The listing builds one solid part. Answer for the finished solid, in the listing's coordinates (mm). A direction names the side the tool comes from. Coordinates: 2 decimals unless noted, no trailing zeros. Order: outer loops, then holes, each group sorted by start corner. A loop starts at its lowest first (then second) coordinate and runs counter-clockwise, first axis right, second up. Notation, with made-up numbers: (-12.5, -8) -> (40.5, -8) arc R22 ccw to (40.5, 18) -> close; hole circle Ø4 at (52.5, -10.5). An arc over 180 degrees is marked (long way). Return JSON: item names as keys, results as strings.
```python
from build123d import *

# Parameters (mm, degrees)
SKETCH1_W           = 300
SKETCH1_H           = 300
SKETCH1_W_2         = 287.3
SKETCH1_H_2         = 287.3
BOSS_EXTRUDE1_DEPTH = 39.8272
CUT_EXTRUDE1_REACH  = 339.766
SKETCH3_W           = 9.414604459
SKETCH3_H           = 11.065164
SKETCH3_W_2         = 16.002
SKETCH3_H_2         = 13.335
SKETCH3_W_3         = 15.3
SKETCH3_H_3         = 12.7
SKETCH3_W_4         = 9
SKETCH3_H_4         = 11


with BuildPart() as part:
    # Sketch1 → Boss-Extrude1 (new body)
    with BuildSketch(Plane(origin=(0, 0, 0), x_dir=(1, 0, 0), z_dir=(0, 1, 0))):
        Rectangle(SKETCH1_W, SKETCH1_H)
        Rectangle(SKETCH1_W_2, SKETCH1_H_2, mode=Mode.SUBTRACT)
    extrude(amount=BOSS_EXTRUDE1_DEPTH)

    # Sketch3 → Cut-Extrude1 (cut, up to next)
    with BuildSketch(Plane(origin=(0, 0, -150), x_dir=(-1, 0, 0), z_dir=(0, 0, -1)), mode=Mode.PRIVATE) as cut_extrude1_sk1:
        with Locations((-111.859321897, 7.773371258)):
            Rectangle(SKETCH3_W, SKETCH3_H)
    cut_extrude1_tool1 = extrude(cut_extrude1_sk1.sketch, amount=-CUT_EXTRUDE1_REACH, mode=Mode.PRIVATE) & part.part
    # Sketch3 → Cut-Extrude1 (cut, up to next)
    with BuildSketch(Plane(origin=(0, 0, -150), x_dir=(-1, 0, 0), z_dir=(0, 0, -1)), mode=Mode.PRIVATE) as cut_extrude1_sk2:
        with Locations((-91.547624126, 6.5913)):
            Rectangle(SKETCH3_W_2, SKETCH3_H_2)
    cut_extrude1_tool2 = extrude(cut_extrude1_sk2.sketch, amount=-CUT_EXTRUDE1_REACH, mode=Mode.PRIVATE) & part.part
    # Sketch3 → Cut-Extrude1 (cut, up to next)
    with BuildSketch(Plane(origin=(0, 0, -150), x_dir=(-1, 0, 0), z_dir=(0, 0, -1)), mode=Mode.PRIVATE) as cut_extrude1_sk3:
        with Locations((-38.618448478, 7.9248)):
            Rectangle(SKETCH3_W_3, SKETCH3_H_3)
    cut_extrude1_tool3 = extrude(cut_extrude1_sk3.sketch, amount=-CUT_EXTRUDE1_REACH, mode=Mode.PRIVATE) & part.part
    # Sketch3 → Cut-Extrude1 (cut, up to next)
    with BuildSketch(Plane(origin=(0, 0, -150), x_dir=(-1, 0, 0), z_dir=(0, 0, -1)), mode=Mode.PRIVATE) as cut_extrude1_sk4:
        with Locations((-18.092571078, 7.9248)):
            Rectangle(SKETCH3_W_3, SKETCH3_H_3)
    cut_extrude1_tool4 = extrude(cut_extrude1_sk4.sketch, amount=-CUT_EXTRUDE1_REACH, mode=Mode.PRIVATE) & part.part
    # Sketch3 → Cut-Extrude1 (cut, up to next)
    with BuildSketch(Plane(origin=(0, 0, -150), x_dir=(-1, 0, 0), z_dir=(0, 0, -1)), mode=Mode.PRIVATE) as cut_extrude1_sk5:
        with Locations((6.757428922, 7.1748)):
            Rectangle(SKETCH3_W_4, SKETCH3_H_4)
    cut_extrude1_tool5 = extrude(cut_extrude1_sk5.sketch, amount=-CUT_EXTRUDE1_REACH, mode=Mode.PRIVATE) & part.part
    # Sketch3 → Cut-Extrude1 (cut, up to next)
    with BuildSketch(Plane(origin=(0, 0, -150), x_dir=(-1, 0, 0), z_dir=(0, 0, -1)), mode=Mode.PRIVATE) as cut_extrude1_sk6:
        with Locations((28.457428922, 7.1748)):
            Rectangle(SKETCH3_W_4, SKETCH3_H_4)
    cut_extrude1_tool6 = extrude(cut_extrude1_sk6.sketch, amount=-CUT_EXTRUDE1_REACH, mode=Mode.PRIVATE) & part.part
    add(cut_extrude1_tool1.solids().sort_by_distance((111.859322, 7.773371, -150))[0], mode=Mode.SUBTRACT)
    add(cut_extrude1_tool2.solids().sort_by_distance((91.547624, 6.5913, -150))[0], mode=Mode.SUBTRACT)
    add(cut_extrude1_tool3.solids().sort_by_distance((38.618448, 7.9248, -150))[0], mode=Mode.SUBTRACT)
    add(cut_extrude1_tool4.solids().sort_by_distance((18.092571, 7.9248, -150))[0], mode=Mode.SUBTRACT)
    add(cut_extrude1_tool5.solids().sort_by_distance((-6.757429, 7.1748, -150))[0], mode=Mode.SUBTRACT)
    add(cut_extrude1_tool6.solids().sort_by_distance((-28.457429, 7.1748, -150))[0], mode=Mode.SUBTRACT)


solid = part.part
```
Item 1: A flat-ended cylindrical pin translates along its axis: pin 1 (7 mm diameter, centred on x = -28, z = -147.5, fed in from -Y). Find the tip coordinate at first contact, or state that the pin passes through.
Answer list:
{"pin 1": "y = 0"}
Item 2: Find the intervals of material crossed by probe 1 along X at (y, z) = (6.5, 53.5); probe 2 along Z at (x, y) = (89.5, 11), in increasing order.
Answer list:
{"probe 1": "-150 to -143.65, 143.65 to 150", "probe 2": "143.65 to 150"}
Item 3: The part is cut by section C-C on y = 30. Determine the outline of the cut face in (x, z), plus the area to 3 significant figures.
Answer list:
{"outline": "(-150, -150) -> (150, -150) -> (150, 150) -> (-150, 150) -> close; hole (-143.65, -143.65) -> (143.65, -143.65) -> (143.65, 143.65) -> (-143.65, 143.65) -> close", "area": "7,460 mm2"}
Item 4: The part is cut by section A-A on z = -66. Determine the outline of the cut face in (x, y), plus the area to 3 significant figures.
Answer list:
{"outline": "(-150, 0) -> (-143.65, 0) -> (-143.65, 39.83) -> (-150, 39.83) -> close; (143.65, 0) -> (150, 0) -> (150, 39.83) -> (143.65, 39.83) -> close", "area": "506 mm2"}
Item 5: Determine the mould class of faces 1 (the flat face through (-2, 20, 150)), 2 (the flat face through (-2, 20, -143.65)), 3 (the flat face through (150, 20, 2)) for opening direction Z: pulls with the +Z half, pulls with the -Z half, needs draft (parallel to the pull), parting line crosses it, or undercut.
Answer list:
{"face 1": "pulls with the +Z half", "face 2": "undercut", "face 3": "needs draft"}
Item 6: Which of the six approach directions +Z, -Z, +X, -X, +Y, -Y give full straight-line access (tool end or side, diameter ignored) to faces 4 (the flat face through (-2, 20, 143.65)), 5 (the flat face through (-150, 20, 2))?
Answer list:
{"face 4": "+Y, -Y", "face 5": "+Z, -Z, -X, +Y, -Y"}
Item 7: The part is cut by section D-D on x = 55.5. Determine the outline of the cut face in (y, z), plus the area to 3 significant figures.
Answer list:
{"outline": "(0, -150) -> (39.83, -150) -> (39.83, -143.65) -> (0, -143.65) -> close; (0, 143.65) -> (39.83, 143.65) -> (39.83, 150) -> (0, 150) -> close", "area": "506 mm2"}
Item 8: The part is cut by section B-B on y = 7. Count the separate pieces of the cut face and the enclosed holes in it, plus the area to 3 significant figures.
Answer list:
{"separate pieces": "6", "enclosed holes": "0", "area": "6,990 mm2"}
